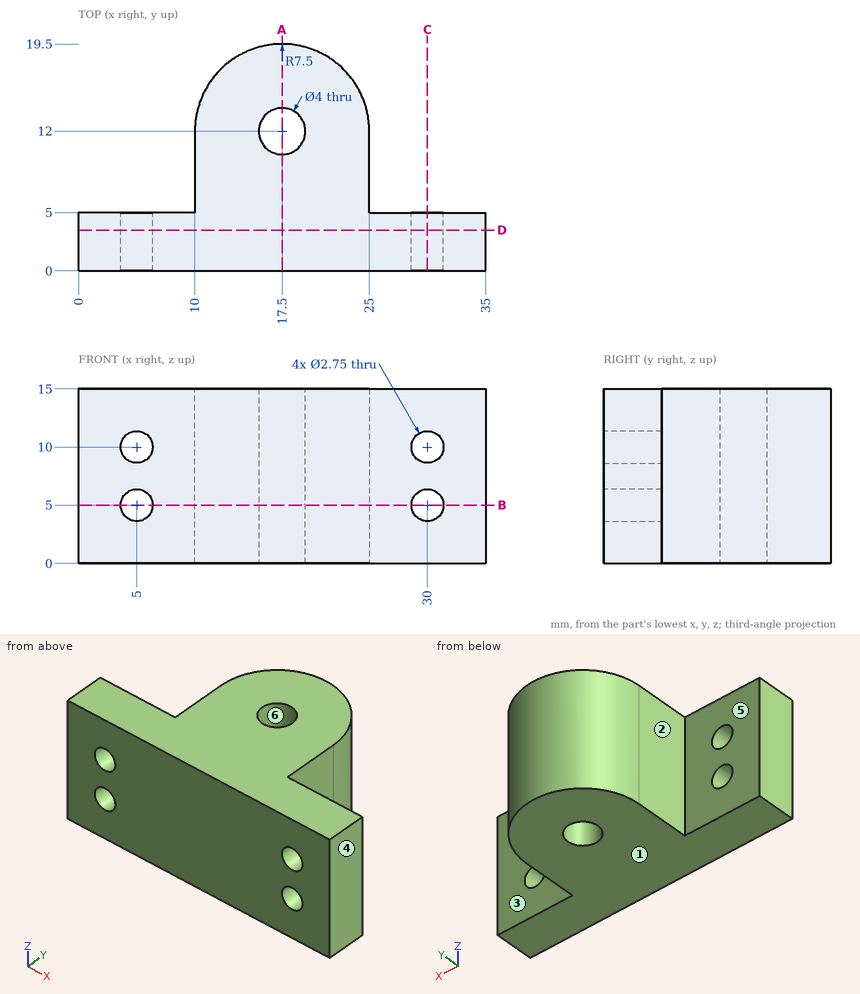
Check sheet for the drawn part. Datum: minimum x, y, z corner. Units: mm. A direction names the side the tool comes from. Give positions to 0.01 mm unless a question says otherwise; leave off trailing zeros. Order: outer loops, then holes, each group sorted by start corner. A loop starts at its lowest first (then second) coordinate and runs counter-clockwise, first axis right, second up.
1. Sectioned sample at C-C (x = 30). Record the boundary of the cut face in (y, z) (3 decimals), then the cut area to 3 significant figures.
Completed:
outline: (0, 0) - (5, 0) - (5, 3.625) - (0, 3.625) - close; (0, 6.375) - (5, 6.375) - (5, 8.625) - (0, 8.625) - close; (0, 11.375) - (5, 11.375) - (5, 15) - (0, 15) - close
area: 47.5 mm2
2. Sectioned sample at A-A (x = 17.5). Record the boundary of the cut face in (y, z).
Completed:
outline: (0, 0) - (10, 0) - (10, 15) - (0, 15) - close; (14, 0) - (19.5, 0) - (19.5, 15) - (14, 15) - close
3. Draft check along X on the marked faces 4, 5 and 6. Enter one of: pulls with the +X half, pulls with the -X half, needs draft (parallel to the pull), parting line crosses it, or undercut.
Completed:
face 4: pulls with the +X half
face 5: needs draft
face 6: undercut
4. Sectioned sample at B-B (z = 5). Record the boundary of the cut face in (x, y) (3 decimals), then the cut area to 3 significant figures.
Completed:
outline: (0, 0) - (3.625, 0) - (3.625, 5) - (0, 5) - close; (6.375, 0) - (28.625, 0) - (28.625, 5) - (25, 5) - (25, 12) arc R7.5 ccw to (10, 12) - (10, 5) - (6.375, 5) - close; (31.375, 0) - (35, 0) - (35, 5) - (31.375, 5) - close; hole circle Ø4 at (17.5, 12)
area: 328 mm2
5. Scan lines: line 1 (X direction, y = 2, z = 10) (3 decimals); line 2 (Z direction, x = 5, y = 1.8) (3 decimals); line 3 (Y direction, x = 17.5, z = 6.5). Record each from-to range of solid material in increasing order.
Completed:
line 1: x = 0 to 3.625, 6.375 to 28.625, 31.375 to 35
line 2: z = 0 to 3.625, 6.375 to 8.625, 11.375 to 15
line 3: y = 0 to 10, 14 to 19.5
6. Sectioned sample at D-D (y = 3.5). Record the boundary of the cut face in (x, z) (3 decimals).
Completed:
outline: (0, 0) - (35, 0) - (35, 15) - (0, 15) - close; hole circle Ø2.75 at (5, 5); hole circle Ø2.75 at (5, 10); hole circle Ø2.75 at (30, 5); hole circle Ø2.75 at (30, 10)
7. Access from +Z, -Z, +X, -X, +Y, -Y to the whole of each face (thin tool, end or side, straight path). Record for the marked faces 1, 2 and 3.
Completed:
face 1: -Z, +X, -X, +Y, -Y
face 2: +Z, -Z, -X, +Y
face 3: +Z, -Z, +X, +Y
8. Depth check by flat-ended pin: pin 1 (3 mm diameter, centred on x = 3.5, z = 10.5, fed in from +Y); pin 2 (3 mm diameter, centred on y = 15, z = 11, fed in from -X); pin 3 (8 mm diameter, centred on y = 13, z = 8, fed in from +X). Enter the tip coordinate at first touch or a pass-through.
Completed:
pin 1: stops at y = 5
pin 2: stops at x = 10.15
pin 3: stops at x = 25
